Design review of the part built by this model. Coordinates are the model's own, in mm. Face numbers are marked on the shaded views. A direction names the side the tool comes from. Round coordinates to 2 decimals unless told otherwise and drop trailing zeros. Loops run counter-clockwise (first coordinate to the right, second up) from the corner with the lowest first, then second, coordinate; pieces in that order, holes last. Notation, with made-up numbers: (86, 16.25) -> (129, 16.25) arc R32 cw to (129, 47.25) -> close; hole circle Ø10 at (29.5, 35.25). An arc over 180 degrees is marked (long way). Write each question's results on one line, items separated by ' | '. Start each with the question number.
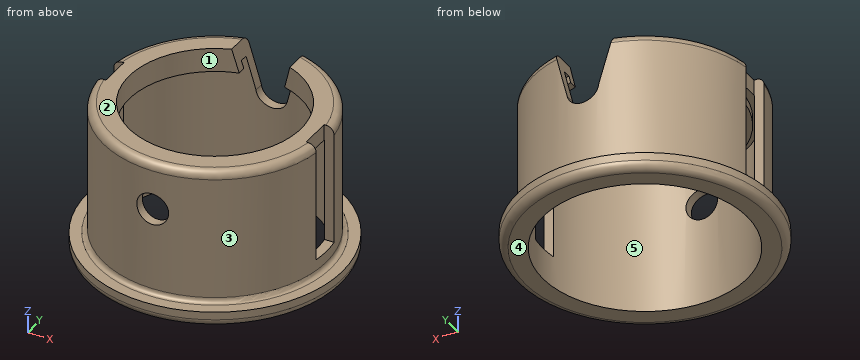
from build123d import *

# Parameters (mm, degrees)
BOX004_W               = 20
BOX004_H               = 20
BOX004_DEPTH           = 80
BOX003_W               = 20
BOX003_H               = 20
BOX003_DEPTH           = 80
BOX002_W               = 10
BOX002_H               = 25
BOX002_DEPTH           = 35
BOX002_PITCH_ANGLE     = -15
BOX001_W               = 10
BOX001_H               = 25
BOX001_DEPTH           = 35
BOX001_PITCH_ANGLE     = 15
BOX_W                  = 20
BOX_H                  = 25
BOX_DEPTH              = 35
CYLINDER005_R          = 10
CYLINDER005_DEPTH      = 180
CYLINDER005_ROLL_ANGLE = 90
CYLINDER004_R          = 54
CYLINDER004_DEPTH      = 100
CYLINDER003_R          = 59
CYLINDER003_DEPTH      = 10
CYLINDER002_R          = 64
CYLINDER002_DEPTH      = 85
CYLINDER001_R          = 70
CYLINDER001_DEPTH      = 90
CYLINDER_R             = 80
CYLINDER_DEPTH         = 10
FILLET_R               = 3
FILLET001_R            = 5
FILLET002_R            = 5


with BuildPart() as tab_cut_l:
    # Box004 → Box004 (new body)
    with BuildSketch(Plane(origin=(-83, -10, 20), x_dir=(1, 0, 0), z_dir=(0, 0, 1))):
        with Locations((10, 10)):
            Rectangle(BOX004_W, BOX004_H)
    extrude(amount=BOX004_DEPTH)


with BuildPart() as tab_cut_r:
    # Box003 → Box003 (new body)
    with BuildSketch(Plane(origin=(63, -10, 20), x_dir=(1, 0, 0), z_dir=(0, 0, 1))):
        with Locations((10, 10)):
            Rectangle(BOX003_W, BOX003_H)
    extrude(amount=BOX003_DEPTH)


with BuildPart() as cube001:
    # Box002 → Box002 (new body)
    with BuildSketch(Plane.XY):
        with Locations((5, 12.5)):
            Rectangle(BOX002_W, BOX002_H)
    extrude(amount=BOX002_DEPTH)


with BuildPart() as cube001_1:
    # Box002 pitch: moved
    add(cube001.part.rotate(Axis((0, 0, 0), (0, 1, 0)), BOX002_PITCH_ANGLE))


with BuildPart() as cube001_2:
    # Box002 placement: moved
    add(cube001_1.part.moved(Location((-9.95, 48, 64))))


with BuildPart() as cube:
    # Box001 → Box001 (new body)
    with BuildSketch(Plane.XY):
        with Locations((5, 12.5)):
            Rectangle(BOX001_W, BOX001_H)
    extrude(amount=BOX001_DEPTH)


with BuildPart() as cube_1:
    # Box001 pitch: moved
    add(cube.part.rotate(Axis((0, 0, 0), (0, 1, 0)), BOX001_PITCH_ANGLE))


with BuildPart() as cube_2:
    # Box001 placement: moved
    add(cube_1.part.moved(Location((0, 48, 65))))


with BuildPart() as bearing_slot:
    # Box → Box (new body)
    with BuildSketch(Plane(origin=(-10, 48, 65), x_dir=(1, 0, 0), z_dir=(0, 0, 1))):
        with Locations((10, 12.5)):
            Rectangle(BOX_W, BOX_H)
    extrude(amount=BOX_DEPTH)


with BuildPart() as bearing_holes:
    # Cylinder005 → Cylinder005 (new body)
    with BuildSketch(Plane.XY):
        Circle(CYLINDER005_R)
    extrude(amount=CYLINDER005_DEPTH)


with BuildPart() as bearing_holes_1:
    # Cylinder005 roll: moved
    add(bearing_holes.part.rotate(Axis((0, 0, 0), (1, 0, 0)), CYLINDER005_ROLL_ANGLE))


with BuildPart() as bearing_holes_2:
    # Cylinder005 placement: moved
    add(bearing_holes_1.part.moved(Location((0, 90, 65))))


with BuildPart() as through_hole:
    # Cylinder004 → Cylinder004 (new body)
    with BuildSketch(Plane.XY):
        Circle(CYLINDER004_R)
    extrude(amount=CYLINDER004_DEPTH)


with BuildPart() as inner_lip:
    # Cylinder003 → Cylinder003 (new body)
    with BuildSketch(Plane.XY.offset(80)):
        Circle(CYLINDER003_R)
    extrude(amount=CYLINDER003_DEPTH)


with BuildPart() as inner_hole:
    # Cylinder002 → Cylinder002 (new body)
    with BuildSketch(Plane.XY):
        Circle(CYLINDER002_R)
    extrude(amount=CYLINDER002_DEPTH)


with BuildPart() as body_cylinder:
    # Cylinder001 → Cylinder001 (new body)
    with BuildSketch(Plane.XY.offset(5)):
        Circle(CYLINDER001_R)
    extrude(amount=CYLINDER001_DEPTH)


with BuildPart() as cut007:
    # Cylinder → Cylinder (new body)
    with BuildSketch(Plane.XY):
        Circle(CYLINDER_R)
    extrude(amount=CYLINDER_DEPTH)

    # Fusion: union Body_Cylinder
    add(body_cylinder.part)

    # Cut: cut Inner_Hole
    add(inner_hole.part, mode=Mode.SUBTRACT)

    # Fusion001: union Inner_Lip
    add(inner_lip.part)

    # Cut001: cut Through_Hole
    add(through_hole.part, mode=Mode.SUBTRACT)

    # Fillet
    fillet_edges = [cut007.edges().sort_by_distance(p)[0] for p in [
        (-70, 0, 10),
    ]]
    fillet(fillet_edges, radius=FILLET_R)

    # Fillet001
    fillet001_edges = [cut007.edges().sort_by_distance(p)[0] for p in [
        (-80, 0, 0),
    ]]
    fillet(fillet001_edges, radius=FILLET001_R)

    # Fillet002
    fillet002_edges = [cut007.edges().sort_by_distance(p)[0] for p in [
        (-70, 0, 95),
    ]]
    fillet(fillet002_edges, radius=FILLET002_R)

    # Cut002: cut Bearing_Holes
    add(bearing_holes_2.part, mode=Mode.SUBTRACT)

    # Cut003: cut Bearing_Slot
    add(bearing_slot.part, mode=Mode.SUBTRACT)

    # Cut004: cut Cube
    add(cube_2.part, mode=Mode.SUBTRACT)

    # Cut005: cut Cube001
    add(cube001_2.part, mode=Mode.SUBTRACT)

    # Cut006: cut Tab_Cut_R
    add(tab_cut_r.part, mode=Mode.SUBTRACT)

    # Cut007: cut Tab_Cut_L
    add(tab_cut_l.part, mode=Mode.SUBTRACT)


solid = cut007.part
1) Take a section at B-B (x = 0). Write out the cut boundary in (y, z), plus the area to 3 significant figures.
2) The part is to be moulded in two halves that separate along Y. For the marked faces 1, 2 and 3, say which applies: +Y half, -Y half, draft (parallel to the pull), parting line (faces both ways), or undercut.
3) For the marked faces 4 and 5, list the 3-axis set-ups (+Z, -Z, +X, -X, +Y, -Y) from which the entire face can be reached by the end or side of a thin tool; tool diameter is ignored.
4) Insertion check: pin 1 (3 mm diameter, centred on x = -66, z = 53, fed in from +Y); pin 2 (5 mm diameter, centred on x = -28, z = 19.5, fed in from +Y); pin 3 (2 mm diameter, centred on y = -46, z = 31, fed in from -X). Each pin has a flat end and moves straight along its axis. Give the tip position at first contact, or say it passes through.
5) Take a section at A-A (y = 0). Write out the cut boundary in (x, z).
6) Take a section at C-C (z = 58). Write out the cut boundary in (x, y).
7) To check wall thickness, follow line 1 (Y direction, x = 0, z = 83.75); line 2 (X direction, y = 0, z = 86); line 3 (Z direction, x = -40, y = -63). State the ranges of each line that lie inside material, in increasing order. Write a range as from..to.
Geometry check:
1) outline: (-80, 5) arc R5 ccw to (-75, 0) -> (-64, 0) -> (-64, 55) -> (-70, 55) -> (-70, 13) arc R3 cw to (-73, 10) -> (-80, 10) -> close; (-70, 75) -> (-64, 75) -> (-64, 85) -> (-59, 85) -> (-59, 80) -> (-54, 80) -> (-54, 95) -> (-65, 95) arc R5 ccw to (-70, 90) -> close; (64, 0) -> (75, 0) arc R5 ccw to (80, 5) -> (80, 10) -> (73, 10) arc R3 cw to (70, 13) -> (70, 55) -> (64, 55) -> close | area: 1,090 mm^2
2) face 1: undercut | face 2: draft | face 3: parting line
3) face 4: -Z, +X, -X, +Y, -Y | face 5: -Z
4) pin 1: stops at y = 27.2 | pin 2: stops at y = 65.19 | pin 3: stops at x = -53.62
5) outline: (-80, 5) arc R5 ccw to (-75, 0) -> (-64, 0) -> (-64, 20) -> (-70, 20) -> (-70, 13) arc R3 cw to (-73, 10) -> (-80, 10) -> close; (-63, 85) -> (-59, 85) -> (-59, 80) -> (-54, 80) -> (-54, 95) -> (-63, 95) -> close; (54, 80) -> (59, 80) -> (59, 85) -> (63, 85) -> (63, 95) -> (54, 95) -> close; (64, 0) -> (75, 0) arc R5 ccw to (80, 5) -> (80, 10) -> (73, 10) arc R3 cw to (70, 13) -> (70, 20) -> (64, 20) -> close
6) outline: (-69.28, -10) arc R70 ccw to (-7.14, -69.63) -> (-7.14, -63.6) arc R64 cw to (-63.21, -10) -> close; (-69.28, 10) -> (-63.21, 10) arc R64 cw to (-7.14, 63.6) -> (-7.14, 69.63) arc R70 ccw to start; (7.14, -69.63) arc R70 ccw to (69.28, -10) -> (63.21, -10) arc R64 cw to (7.14, -63.6) -> close; (7.14, 63.6) arc R64 cw to (63.21, 10) -> (69.28, 10) arc R70 ccw to (7.14, 69.63) -> close
7) line 1: y = -70..-64, -59..-54 | line 2: x = -63..-54, 54..63 | line 3: z = 0..10
